Job drawing, mm, ordinate dimensions from the low corner. One solid piece. A direction names the side the tool comes from. Give positions to 0.01 mm unless a question says otherwise; leave off trailing zeros. Loops run counter-clockwise (first coordinate to the right, second up) from the corner with the lowest first, then second, coordinate; pieces in that order, holes last. Notation, with made-up numbers: (27, -19.5) - (36, -19.5) arc R28 ccw to (36, 9.5) - close; hole circle Ø10 at (71, 12). An arc over 180 degrees is marked (long way). Use a Markdown table: item, result.
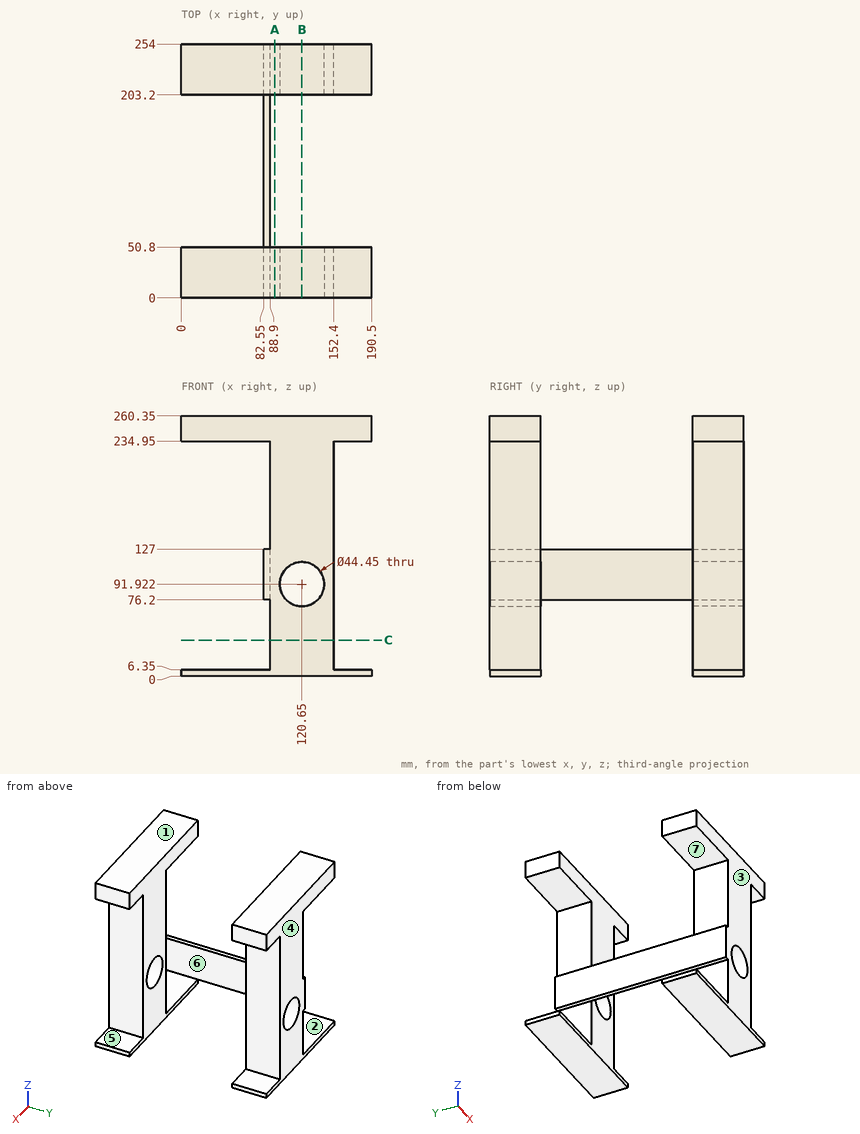
(1) Slice it at A-A, the plane x = 93.5. Write the cut outline in (y, z).
Computed:
| item | result |
|---|---|
| outline | (0, 0) - (50.8, 0) - (50.8, 260.35) - (0, 260.35) - close; (203.2, 0) - (254, 0) - (254, 260.35) - (203.2, 260.35) - close |
(2) Drill centre lines: probe 1 along Y at (x, z) = (119, 127.5); probe 2 along Z at (x, y) = (120, 23); probe 3 along Z at (x, y) = (179, 242). Where is each one in solid material? Low to high. Write a range as [from, to].
Computed:
| item | result |
|---|---|
| probe 1 | [0, 50.8], [203.2, 254] |
| probe 2 | [0, 69.71], [114.14, 260.35] |
| probe 3 | [0, 6.35], [234.95, 260.35] |
(3) Pin check, flat tips, straight feed: P1, Ø15, axis at y = 92, z = 109, coming from the -X side; P2, Ø2, axis at y = 223.5, z = 103, coming from the +X side; P3, Ø2, axis at x = 126.5, y = 217, coming from the -Z side; P4, Ø7, axis at x = 84.5, y = 137.5, coming from the -Z side. Stop position of each tip, or through.
Computed:
| item | result |
|---|---|
| P1 | x = 82.55 |
| P2 | x = 152.4 |
| P3 | z = 0 |
| P4 | z = 76.2 |
(4) Slice it at C-C, the plane z = 36. Write the cut outline in (x, y), plus the area to 3 significant figures.
Computed:
| item | result |
|---|---|
| outline | (88.9, 0) - (152.4, 0) - (152.4, 50.8) - (88.9, 50.8) - close; (88.9, 203.2) - (152.4, 203.2) - (152.4, 254) - (88.9, 254) - close |
| area | 6,450 mm² |
(5) 3-axis set-ups, long thin cutter, end or side, ignore diameter. For the marked faces 4, 5, 6 and 7: which of +Z, -Z, +X, -X, +Y, -Y reach the whole face in a straight line?
Computed:
| item | result |
|---|---|
| face 4 | +Z, -Z, +X, -X, +Y |
| face 5 | +X, +Y, -Y |
| face 6 | +Z, -Z, +X |
| face 7 | -X, +Y, -Y |
(6) Mould opens along Z. For the marked faces 1, 2 and 3 say: pulls with the +Z half, pulls with the -Z half, needs draft (parallel to the pull), parting line crosses it, or undercut.
Computed:
| item | result |
|---|---|
| face 1 | pulls with the +Z half |
| face 2 | undercut |
| face 3 | needs draft |
(7) Slice it at B-B, the plane x = 120.65. Write the cut outline in (y, z), plus the area to 3 significant figures.
Computed:
| item | result |
|---|---|
| outline | (0, 0) - (50.8, 0) - (50.8, 69.7) - (0, 69.7) - close; (0, 114.15) - (50.8, 114.15) - (50.8, 260.35) - (0, 260.35) - close; (203.2, 0) - (254, 0) - (254, 69.7) - (203.2, 69.7) - close; (203.2, 114.15) - (254, 114.15) - (254, 260.35) - (203.2, 260.35) - close |
| area | 21,900 mm² |
